Geometry check sheet. Reference: the model listing, model coordinates, mm. Face numbers are marked on the shaded views. Round coordinates to 2 decimals unless told otherwise and drop trailing zeros. Write each loop counter-clockwise with the first axis right and the second up, starting at its lowest first coordinate (ties: lowest second). Pieces come first, ordered by that corner, then holes. Notation, with made-up numbers: (86.5, 86.5) -> (132.5, 86.5) arc R22 cw to (132.5, 103.5) -> close; hole circle Ø7 at (49.25, -27.75). An arc over 180 degrees is marked (long way). One line per question, with ' | ' between items.
```python
from build123d import *

# Parameters (mm, degrees)
SKETCH1_W                               = 156
SKETCH1_H                               = 314.5
SKETCH1_R                               = 2.55
BOSS_EXTRUDE1_DEPTH                     = 12.7
SKETCH2_R                               = 5.5
CUT_EXTRUDE1_DEPTH                      = 7
M5X0_8_TAPPED_HOLE5_D                   = 4.2
CHAMFER1_SIZE                           = 1
M5X0_8_TAPPED_HOLE3_D                   = 4.2
M5X0_8_TAPPED_HOLE3_DEPTH               = 20.4
M5X0_8_TAPPED_HOLE3_TIP                 = 1.2618073
SKETCH8_W                               = 14
SKETCH8_H                               = 62
CUT_EXTRUDE3_DEPTH                      = 224.909669287
SKETCH9_W                               = 156
SKETCH9_H                               = 20
CUT_EXTRUDE_THIN1_DEPTH                 = 5.5
SKETCH10_R                              = 2.1
BOSS_EXTRUDE2_DEPTH                     = 12.7
FILLET1_R                               = 10
M5X0_8_TAPPED_HOLE2_D                   = 4.2
M5X0_8_TAPPED_HOLE2_CSINK_D             = 5.05
M5X0_8_TAPPED_HOLE2_CSINK_ANGLE         = 90
M6X1_0_TAPPED_HOLE2_D                   = 5
M6X1_0_TAPPED_HOLE2_CSINK_D             = 6.05
M6X1_0_TAPPED_HOLE2_CSINK_ANGLE         = 90
SKETCH16_W                              = 62
SKETCH16_H                              = 27
SKETCH16_H_2                            = 22
CUT_EXTRUDE4_DEPTH                      = 2.3
CBORE_FOR_M5_HEX_HEAD_BOLT1_D           = 5.5
CBORE_FOR_M5_HEX_HEAD_BOLT1_CBORE_D     = 12.24
CBORE_FOR_M5_HEX_HEAD_BOLT1_CBORE_DEPTH = 4.08
M5X0_8_TAPPED_HOLE4_D                   = 4.2
M5X0_8_TAPPED_HOLE4_DEPTH               = 24
M5X0_8_TAPPED_HOLE4_TIP                 = 1.2618073
SKETCH27_R                              = 3
CUT_EXTRUDE5_DEPTH                      = 2.3
FILLET2_R                               = 4


with BuildPart() as part:
    # Sketch1 → Boss-Extrude1 (new body)
    with BuildSketch(Plane.XY):
        with Locations((0, 52.25)):
            Rectangle(SKETCH1_W, SKETCH1_H)
        with Locations((30, -44)):
            Circle(SKETCH1_R, mode=Mode.SUBTRACT)
        with Locations((66, -44)):
            Circle(SKETCH1_R, mode=Mode.SUBTRACT)
        with Locations((30, -76)):
            Circle(SKETCH1_R, mode=Mode.SUBTRACT)
        with Locations((66, -76)):
            Circle(SKETCH1_R, mode=Mode.SUBTRACT)
        with Locations(Location((-66, -44, 0), (0, 0, 180))):
            Circle(SKETCH1_R, mode=Mode.SUBTRACT)
        with Locations(Location((-66, -76, 0), (0, 0, 180))):
            Circle(SKETCH1_R, mode=Mode.SUBTRACT)
        with Locations(Location((-30, -76, 0), (0, 0, 180))):
            Circle(SKETCH1_R, mode=Mode.SUBTRACT)
        with Locations(Location((-30, -44, 0), (0, 0, 180))):
            Circle(SKETCH1_R, mode=Mode.SUBTRACT)
        with Locations(Location((66, 76, 0), (0, 0, 180))):
            Circle(SKETCH1_R, mode=Mode.SUBTRACT)
        with Locations(Location((66, 44, 0), (0, 0, 180))):
            Circle(SKETCH1_R, mode=Mode.SUBTRACT)
        with Locations(Location((30, 76, 0), (0, 0, 180))):
            Circle(SKETCH1_R, mode=Mode.SUBTRACT)
        with Locations(Location((30, 44, 0), (0, 0, 180))):
            Circle(SKETCH1_R, mode=Mode.SUBTRACT)
        with Locations((-30, 76)):
            Circle(SKETCH1_R, mode=Mode.SUBTRACT)
        with Locations((-30, 44)):
            Circle(SKETCH1_R, mode=Mode.SUBTRACT)
        with Locations((-66, 76)):
            Circle(SKETCH1_R, mode=Mode.SUBTRACT)
        with Locations((-66, 44)):
            Circle(SKETCH1_R, mode=Mode.SUBTRACT)
    extrude(amount=BOSS_EXTRUDE1_DEPTH)

    # Sketch2 → Cut-Extrude1 (cut)
    with BuildSketch(Plane.XY.offset(12.7)):
        with Locations((-66, 76)):
            Circle(SKETCH2_R)
        with Locations((-30, 76)):
            Circle(SKETCH2_R)
        with Locations((-66, 44)):
            Circle(SKETCH2_R)
        with Locations((-30, 44)):
            Circle(SKETCH2_R)
        with Locations((30, 76)):
            Circle(SKETCH2_R)
        with Locations((66, 76)):
            Circle(SKETCH2_R)
        with Locations((30, 44)):
            Circle(SKETCH2_R)
        with Locations((66, 44)):
            Circle(SKETCH2_R)
        with Locations((-66, -44)):
            Circle(SKETCH2_R)
        with Locations((-30, -44)):
            Circle(SKETCH2_R)
        with Locations((-66, -76)):
            Circle(SKETCH2_R)
        with Locations((-30, -76)):
            Circle(SKETCH2_R)
        with Locations((30, -76)):
            Circle(SKETCH2_R)
        with Locations((30, -44)):
            Circle(SKETCH2_R)
        with Locations((66, -44)):
            Circle(SKETCH2_R)
        with Locations((66, -76)):
            Circle(SKETCH2_R)
    extrude(amount=-CUT_EXTRUDE1_DEPTH, mode=Mode.SUBTRACT)

    # M5x0.8 Tapped Hole5 (through all)
    with Locations(Plane(origin=(53, 165, 12.7), x_dir=(1, 0, 0), z_dir=(0, 0, 1))):
        with Locations((0, 0), (0, -60), (0, -120), (0, -180), (0, -240), (-106, 0), (-106, -60), (-106, -120), (-106, -180), (-106, -240)):
            Hole(M5X0_8_TAPPED_HOLE5_D / 2)

    # Chamfer1
    chamfer1_edges = [part.edges().sort_by_distance(p)[0] for p in [
        (-50.9, -75, 12.7),
        (-50.9, -15, 12.7),
        (-50.9, 45, 12.7),
        (-50.9, 105, 12.7),
        (-50.9, 165, 12.7),
        (55.1, -75, 12.7),
        (55.1, -15, 12.7),
        (55.1, 45, 12.7),
        (55.1, 105, 12.7),
        (55.1, 165, 12.7),
    ]]
    chamfer(chamfer1_edges, length=CHAMFER1_SIZE)

    # M5x0.8 Tapped Hole3
    with Locations(Plane(origin=(0, 209.5, 0), x_dir=(1, 0, 0), z_dir=(0, 1, 0))):
        with Locations((42, -6.35), (14, -6.35), (-14, -6.35), (-42, -6.35)):
            Hole(M5X0_8_TAPPED_HOLE3_D / 2, depth=M5X0_8_TAPPED_HOLE3_DEPTH)
            with Locations((0, 0, -(M5X0_8_TAPPED_HOLE3_DEPTH + M5X0_8_TAPPED_HOLE3_TIP / 2))):  # 118° drill point
                Cone(0, M5X0_8_TAPPED_HOLE3_D / 2, M5X0_8_TAPPED_HOLE3_TIP, mode=Mode.SUBTRACT)

    # Sketch8 → Cut-Extrude3 (cut, through all)
    with BuildSketch(Plane(origin=(0, 0, 0), x_dir=(-1, 0, 0), z_dir=(0, 0, -1))):
        with Locations((-71, 0)):
            Rectangle(SKETCH8_W, SKETCH8_H)
    extrude(amount=-CUT_EXTRUDE3_DEPTH, mode=Mode.SUBTRACT)

    # Sketch9 → Cut-Extrude-Thin1 (cut)
    with BuildSketch(Plane(origin=(0, 0, 0), x_dir=(-1, 0, 0), z_dir=(0, 0, -1))):
        Rectangle(SKETCH9_W, SKETCH9_H)
    extrude(amount=-CUT_EXTRUDE_THIN1_DEPTH, mode=Mode.SUBTRACT)

    # Sketch10 → Boss-Extrude2 (add)
    # profile 1 of 2: a face of its own
    with BuildSketch(Plane.XY.offset(12.7)):
        Polygon((-121, 28), (-121, 43), (-78, 94.245404482), (-78, 28), align=None)
        with Locations((-111, 34)):
            Circle(SKETCH10_R, mode=Mode.SUBTRACT)
        with Locations((-87, 34)):
            Circle(SKETCH10_R, mode=Mode.SUBTRACT)
    # profile 2 of 2: a face of its own
    with BuildSketch(Plane.XY.offset(12.7)):
        Polygon((-78, -28), (-78, -94.245404482), (-121, -43), (-121, -28), align=None)
        with Locations((-87, -34)):
            Circle(SKETCH10_R, mode=Mode.SUBTRACT)
        with Locations((-111, -34)):
            Circle(SKETCH10_R, mode=Mode.SUBTRACT)
    extrude(amount=-BOSS_EXTRUDE2_DEPTH)

    # Fillet1
    fillet1_edges = [part.edges().sort_by_distance(p)[0] for p in [
        (-78, 94.245404482, 6.35),
        (-121, 43, 6.35),
        (-121, -43, 6.35),
        (-78, -94.245404482, 6.35),
    ]]
    fillet(fillet1_edges, radius=FILLET1_R)

    # M5x0.8 Tapped Hole2 (through all)
    with Locations(Plane.XY.offset(12.7)):
        with Locations((-87, 34), (-111, 34), (-87, -34), (-111, -34)):
            CounterSinkHole(M5X0_8_TAPPED_HOLE2_D / 2, M5X0_8_TAPPED_HOLE2_CSINK_D / 2, counter_sink_angle=M5X0_8_TAPPED_HOLE2_CSINK_ANGLE)

    # M6x1.0 Tapped Hole2 (through all)
    with Locations(Plane.XY.offset(12.7)):
        with Locations((-23, 166.5), (23, 166.5), (-23, 153.5), (23, 153.5), (-23, -95), (23, -95)):
            CounterSinkHole(M6X1_0_TAPPED_HOLE2_D / 2, M6X1_0_TAPPED_HOLE2_CSINK_D / 2, counter_sink_angle=M6X1_0_TAPPED_HOLE2_CSINK_ANGLE)

    # Sketch16 → Cut-Extrude4 (cut)
    with BuildSketch(Plane.XY.offset(12.7)):
        with Locations((0, 160)):
            Rectangle(SKETCH16_W, SKETCH16_H)
        with Locations((0, -95)):
            Rectangle(SKETCH16_W, SKETCH16_H_2)
    extrude(amount=-CUT_EXTRUDE4_DEPTH, mode=Mode.SUBTRACT)

    # CBORE for M5 Hex Head Bolt1 (through all)
    with Locations(Plane.XY.offset(12.7)):
        with Locations((-17.5, 183.65), (0, 183.65), (17.5, 183.65)):
            CounterBoreHole(CBORE_FOR_M5_HEX_HEAD_BOLT1_D / 2, CBORE_FOR_M5_HEX_HEAD_BOLT1_CBORE_D / 2, CBORE_FOR_M5_HEX_HEAD_BOLT1_CBORE_DEPTH)

    # M5x0.8 Tapped Hole4
    with Locations(Plane(origin=(78, 0, 0), x_dir=(0, 0, -1), z_dir=(1, 0, 0))):
        with Locations((-6.35, 60)):
            Hole(M5X0_8_TAPPED_HOLE4_D / 2, depth=M5X0_8_TAPPED_HOLE4_DEPTH)
            with Locations((0, 0, -(M5X0_8_TAPPED_HOLE4_DEPTH + M5X0_8_TAPPED_HOLE4_TIP / 2))):  # 118° drill point
                Cone(0, M5X0_8_TAPPED_HOLE4_D / 2, M5X0_8_TAPPED_HOLE4_TIP, mode=Mode.SUBTRACT)

    # Sketch27 → Cut-Extrude5 (cut)
    with BuildSketch(Plane.XY.offset(10.4)):
        with Locations((-28.978679656, 171.478679656)):
            Circle(SKETCH27_R)
        with Locations((28.978679656, 171.478679656)):
            Circle(SKETCH27_R)
        with Locations((28.978679656, 148.521320344)):
            Circle(SKETCH27_R)
        with Locations((-28.978679656, 148.521320344)):
            Circle(SKETCH27_R)
        with Locations((-28.978679656, -86.021320344)):
            Circle(SKETCH27_R)
        with Locations((28.978679656, -86.021320344)):
            Circle(SKETCH27_R)
    extrude(amount=CUT_EXTRUDE5_DEPTH, mode=Mode.SUBTRACT)

    # Fillet2
    fillet2_edges = [part.edges().sort_by_distance(p)[0] for p in [
        (26.761865711, -84, 11.55),
        (-26.761865711, -84, 11.55),
        (-26.761865711, 173.5, 11.55),
        (26.761865711, 173.5, 11.55),
        (-31, 150.738134289, 11.55),
        (26.761865711, 146.5, 11.55),
        (31, 169.261865711, 11.55),
        (31, 150.738134289, 11.55),
        (-26.761865711, 146.5, 11.55),
        (-31, -88.238134289, 11.55),
        (31, -88.238134289, 11.55),
        (-31, 169.261865711, 11.55),
    ]]
    fillet(fillet2_edges, radius=FILLET2_R)


solid = part.part
```
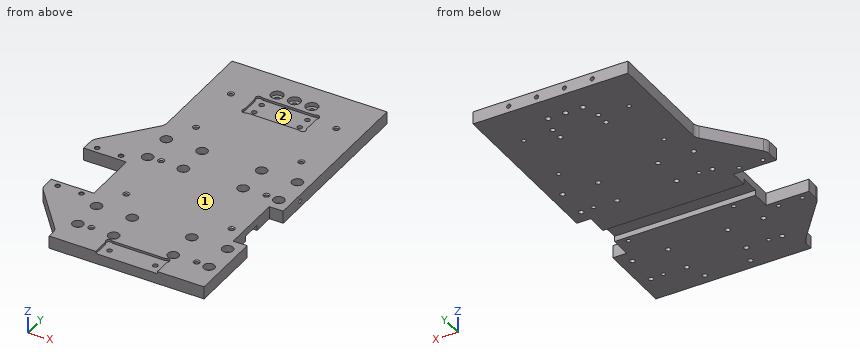
(1) Go/stop test with flat-tipped pins: pin 1 (6 mm diameter, centred on x = 66, y = 44, fed in from -Z); pin 2 (4 mm diameter, centred on y = -4, z = 9.5, fed in from +X); pin 3 (1.5 mm diameter, centred on x = -81, z = 6.5, fed in from +Y). Record where each tip stops, or that it passes through.
Resolved:
pin 1: stops at z = 0 | pin 2: stops at x = 64 | pin 3: stops at y = 91.57
(2) Draft check along X on the marked faces 1 and 2. Enter one of: +X half, -X half, draft (parallel to the pull), parting line (faces both ways), or undercut.
Resolved:
face 1: draft | face 2: undercut
(3) Sectioned sample at B-B on y = -66.5. Record the cut outline in (x, z).
Resolved:
outline: (-101.28, 0) -> (78, 0) -> (78, 12.7) -> (-101.28, 12.7) -> close
(4) Sectioned sample at A-A on y = 0. Record the cut outline in (x, z), then the cut area to 3 significant figures.
Resolved:
outline: (-78, 5.5) -> (64, 5.5) -> (64, 12.7) -> (-78, 12.7) -> close | area: 1,020 mm2
(5) Material ranges on line 1 (Y direction, x = -53, z = 7); line 2 (X direction, y = 153.5, z = 6.75); line 3 (Y direction, x = -66, z = 7.5), recorded low to high.
Resolved:
line 1: y = -105 to -77.1, -72.9 to -17.1, -12.9 to 42.9, 47.1 to 102.9, 107.1 to 162.9, 167.1 to 209.5 | line 2: x = -78 to -25.5, -20.5 to 20.5, 25.5 to 78 | line 3: y = -105 to -81.5, -70.5 to -49.5, -38.5 to 38.5, 49.5 to 70.5, 81.5 to 209.5
